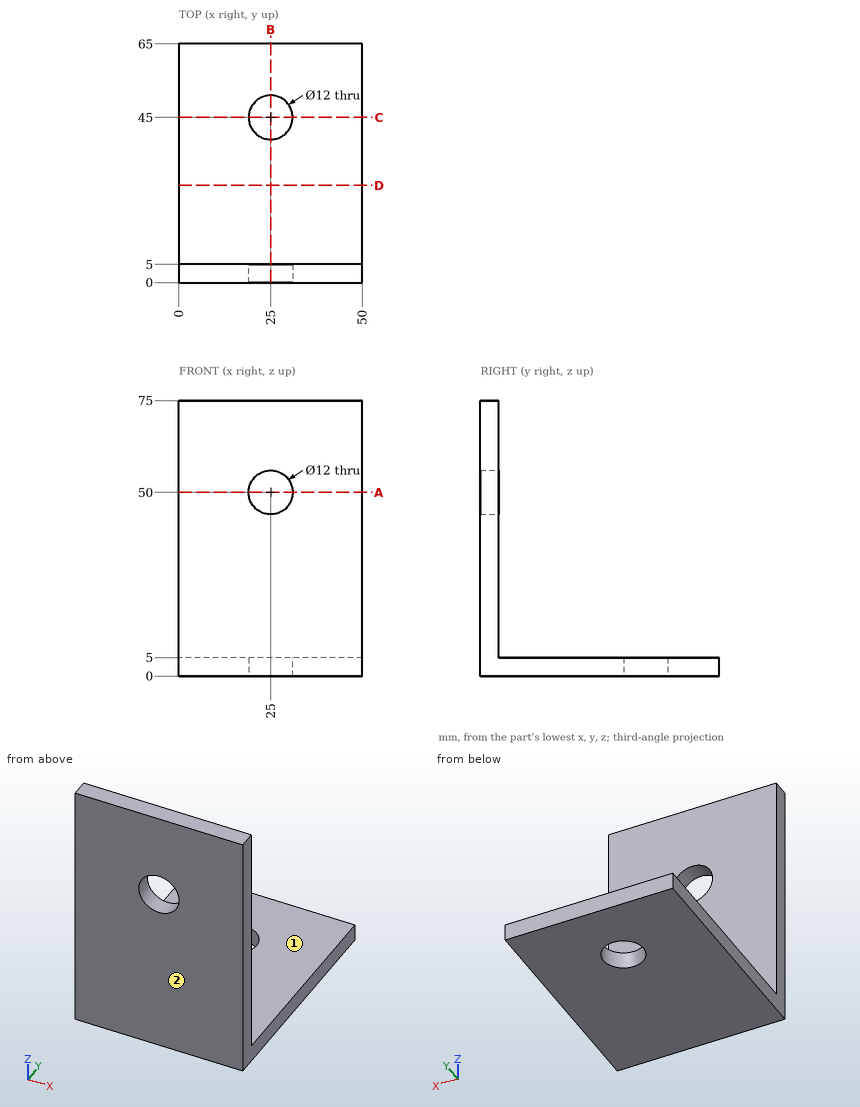
Drawing for the job (mm, zero at the part's lowest x, y, z). A direction names the side the tool comes from. Give positions to 0.01 mm unless a question says otherwise; leave off trailing zeros. Loops run counter-clockwise (first coordinate to the right, second up) from the corner with the lowest first, then second, coordinate; pieces in that order, holes last. Notation, with made-up numbers: (52, -10.5) - (92, -10.5) arc R30 cw to (92, 18.5) - close; hole circle Ø10 at (-13, 88). An arc over 180 degrees is marked (long way). Write item = value, one per line. Start each with the question number.
1) Band-saw the part on B-B on x = 25. Give the cut face in (y, z), plus the area to 3 significant figures.
2) Drop flat-ended pins along their axis: pin 1 Ø8 at (x, y) = (33.5, 24) entering from -Z; pin 2 Ø6 at (x, y) = (30, 23.5) entering from +Z; pin 3 Ø8 at (x, z) = (16.5, 16.5) entering from +Y. Give the stop position or say it passes through.
3) Probe probe 1 along X at (y, z) = (2.4, 50); probe 2 along Y at (x, z) = (26.5, 58); probe 3 along Y at (x, z) = (25, 1.35). List the from-to ranges inside material, lowest first. Write a range as from..to.
4) Band-saw the part on A-A on z = 50. Give the cut face in (x, y), plus the area to 3 significant figures.
5) Tool access for the marked faces 1 and 2: list every direction of +Z, -Z, +X, -X, +Y, -Y with a clear straight run to the whole face (end or side of a thin tool).
6) Band-saw the part on D-D on y = 26.5. Give the cut face in (x, z).
Final values:
q1.outline = (0, 0) - (39, 0) - (39, 5) - (5, 5) - (5, 44) - (0, 44) - close; (0, 56) - (5, 56) - (5, 75) - (0, 75) - close; (51, 0) - (65, 0) - (65, 5) - (51, 5) - close
q1.area = 555 mm²
q2.pin_1 = 0
q2.pin_2 = 5
q2.pin_3 = 5
q3.probe_1 = 0..19, 31..50
q3.probe_2 = 0..5
q3.probe_3 = 0..39, 51..65
q4.outline = (0, 0) - (19, 0) - (19, 5) - (0, 5) - close; (31, 0) - (50, 0) - (50, 5) - (31, 5) - close
q4.area = 190 mm²
q5.face_1 = +Z, +X, -X, +Y
q5.face_2 = +Z, -Z, +X, -X, -Y
q6.outline = (0, 0) - (50, 0) - (50, 5) - (0, 5) - close
